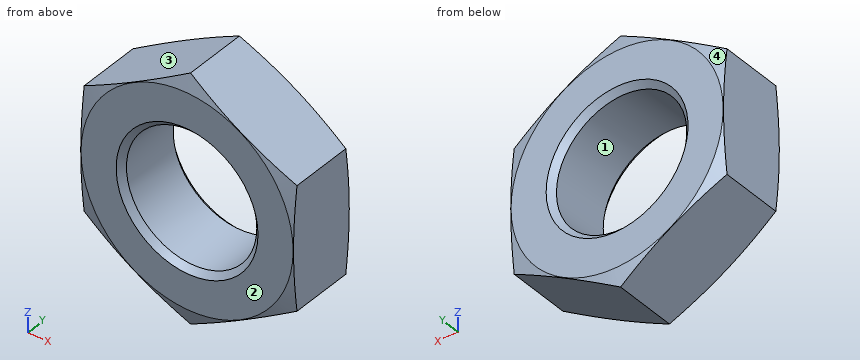
Autodesk Inventor part; units mm, degrees
ref_plane "2CYL_XY" through (0, -5, 0) normal (0, 1, 0) x (1, 0, 0)
ref_plane "2CYL_YZ" through (0, -5, 0) normal (1, 0, 0) x (0, 0, -1)
ref_plane "2CYL_ZX" through (0, -5, 0) normal (0, 0, -1) x (0, 1, 0)
sketch "Sketch_1" plane through (0, 0, 0) normal (0, 0, 1) x (1, 0, 0)
  line L0 (0, -10) -> (0, 0)
  line L1 (0, 0) -> (14.95, 0)
  line L2 (14.95, 0) -> (33.6103, -5)
  line L3 (33.6103, -5) -> (14.95, -10)
  line L4 (14.95, -10) -> (0, -10)
  line L5 (0, -10) -> (0, 0)
revolve "Revolution1" add sketch "Sketch_1" angle 360 about axis through (0, -10, 0) along (0, 1, 0)
sketch "Sketch_2" plane through (0, 0, 0) normal (0, 1, 0) x (-1, 0, 0)
  line L0 (60, -60) -> (60, 60)
  line L1 (60, 60) -> (-60, 60)
  line L2 (-60, 60) -> (-60, -60)
  line L3 (-60, -60) -> (60, -60)
  line L4 (15, 8.6603) -> (0, 17.3205)
  line L5 (0, 17.3205) -> (-15, 8.6603)
  line L6 (-15, 8.6603) -> (-15, -8.6603)
  line L7 (-15, -8.6603) -> (0, -17.3205)
  line L8 (0, -17.3205) -> (15, -8.6603)
  line L9 (15, -8.6603) -> (15, 8.6603)
extrude "Extrusion1" cut sketch "Sketch_2" along normal mid plane 22
sketch "Sketch_3" plane through (0, 0, 0) normal (0, 0, 1) x (1, 0, 0)
  line L0 (0, -10) -> (0, 0)
  line L1 (0, 0) -> (10, 0)
  line L2 (10, 0) -> (9.188, -0.812)
  line L3 (9.188, -0.812) -> (9.188, -9.188)
  line L4 (9.188, -9.188) -> (10, -10)
  line L5 (10, -10) -> (0, -10)
  line L6 (0, -10) -> (0, 0)
revolve "Revolution2" cut sketch "Sketch_3" angle 360 about axis through (0, -10, 0) along (0, -1, 0)
thread "Thread1"
ref_plane "2CYL_XY" through (0, -5, 0) normal (0, 1, 0) x (1, 0, 0)
ref_plane "2CYL_YZ" through (0, -5, 0) normal (1, 0, 0) x (0, 0, -1)
ref_plane "2CYL_ZX" through (0, -5, 0) normal (0, 0, -1) x (0, 1, 0)
ref_plane "din439b_punkt_XY" through (0, 0, 0) normal (0, 1, 0) x (1, 0, 0)
ref_plane "din439b_punkt_YZ" through (0, 0, 0) normal (1, 0, 0) x (0, 0, -1)
ref_plane "din439b_punkt_ZX" through (0, 0, 0) normal (0, 0, -1) x (0, 1, 0)
properties part number "DIN-439-B - M20x1.5(F)"
Model file for the job. Use its own axes, mm. Face numbers are marked on the shaded views. Coordinates: 2 decimals unless noted, no trailing zeros. Order: outer loops, then holes, each group sorted by start corner. A loop starts at its lowest first (then second) coordinate and runs counter-clockwise, first axis right, second up. Notation, with made-up numbers: (-23, 20.5) - (12, 20.5) arc R3 cw to (12, 24.5) - close; hole circle Ø7 at (-38.5, 16.25). An arc over 180 degrees is marked (long way). Return JSON: item names as keys, results as strings. Group by question number.
1) Saw through at A-A, the plane z = 0. Write the cut outline in (x, y), plus the area to 3 significant figures.
2) Saw through at B-B, the plane y = -8.25. Write the cut outline in (x, z), plus the area to 3 significant figures.
3) Mould opens along X. For the marked faces 1, 2, 3 and 4 say: released by +X, released by -X, zero draft, split by the parting line, or undercut.
4) Probe line 1 (Z direction, x = 0, y = -5); line 2 (X direction, y = -5.5, z = 8); line 3 (X direction, y = -7.25, z = 4). List the from-to ranges inside material, lowest first. Write a range as from..to.
5) Flat gauge pins, fed straight in: P1, Ø6, axis at x = -11.5, y = -5, coming from the +Z side; P2, Ø6, axis at x = -8.5, y = -7, coming from the +Z side; P3, Ø4, axis at x = 7.5, z = -5, coming from the +Y side; P4, Ø1, axis at y = -6, z = -10, coming from the -X side. Where does each tip first touch, or does it go through?
Values found:
{
 "1": {"outline": "(-15, -9.99) - (-14.95, -10) - (-10, -10) - (-9.19, -9.19) - (-9.19, -0.81) - (-10, 0) - (-14.95, 0) - (-15, -0.01) - close; (9.19, -9.19) - (10, -10) - (14.95, -10) - (15, -9.99) - (15, -0.01) - (14.95, 0) - (10, 0) - (9.19, -0.81) - close", "area": "115 mm²"},
 "2": {"outline": "(-15, -8.66) - (0, -17.32) - (15, -8.66) - (15, 8.66) - (0, 17.32) - (-15, 8.66) - close; hole circle Ø18.38 at (0, 0)", "area": "514 mm²"},
 "3": {"face 1": "undercut", "face 2": "zero draft", "face 3": "released by -X", "face 4": "split by the parting line"},
 "4": {"line 1": "z = -17.32..-9.19, 9.19..17.32", "line 2": "x = -15..-4.52, 4.52..15", "line 3": "x = -15..-8.27, 8.27..15"},
 "5": {"P1": "stops at z = 12.41", "P2": "stops at z = 14.15", "P3": "stops at y = 0", "P4": "stops at x = -13.55"}
}
